Check sheet for the modelled part. Datum: model origin and axes. Units: mm. A direction names the side the tool comes from. Coordinates: 2 decimals unless noted, no trailing zeros. Loops run counter-clockwise (first coordinate to the right, second up) from the corner with the lowest first, then second, coordinate; pieces in that order, holes last. Notation, with made-up numbers: M 47,52 L 94,52 A12 cw 94,56 Z; hole C 41,21 d10. An arc over 180 degrees is marked long. Use CSV: the item, a comma, the result in double quotes. Start each with the question number.
(1) Section check C-C on y = -7.5. Record the cut outline in (x, z), and give its area (3 significant figures).
(2) Section check B-B on z = 33.5. Record the cut outline in (x, y), and give its area (3 significant figures).
(3) Set-up check for faces 1 (the flat face through (-105, -25.4, 26)), 2 (the flat face through (-90.02, -50.98, 14.5)), 3 (the flat face through (-2, -63.5, 15)): record each of +Z, -Z, +X, -X, +Y, -Y from which the full face is reachable in a straight line by a thin tool's end or side.
(4) Scan lines: line 1 (Y direction, x = -68, z = 31); line 2 (X direction, y = -41, z = 22.5); line 3 (X direction, y = -54.5, z = 24). Record each from-to range of solid material in increasing order.
(5) Section check A-A on x = -65. Record the cut outline in (y, z).
(6) Go/stop test with flat-tipped pins: pin 1 Ø1.5 at (x, z) = (-30.5, 15.5) entering from +Y; pin 2 Ø8 at (x, y) = (-94, -9) entering from +Z. Record where each tip stops, or that it passes through.
from build123d import *

# Parameters (mm, degrees)
F0_W     = 203.2
F0_H     = 50.8
F1_DEPTH = 63.5
F3_DEPTH = 25.4
F5_DEPTH = 25.4


with BuildPart() as f1:
    # F0 (on Front) → F1 (new body)
    with BuildSketch(Plane.XZ):
        with Locations((-22.86, 14.851971)):
            Rectangle(F0_W, F0_H)
    extrude(amount=F1_DEPTH)

    # F2 (on face) → F3 (cut)
    with BuildSketch(Plane.XZ.offset(63.5)):
        Polygon((-124.46, 40.251971), (-124.46, -10.548029), (-54.61, 40.251971), align=None)
    extrude(amount=-F3_DEPTH, mode=Mode.SUBTRACT)

    # F4 (on face) → F5 (cut)
    with BuildSketch(Plane(origin=(0, 0, 0), x_dir=(-1, 0, 0), z_dir=(0, 1, 0))):
        Polygon((54.61, 40.251971), (124.46, -10.548029), (124.46, 40.251971), align=None)
    extrude(amount=-F5_DEPTH, mode=Mode.SUBTRACT)


solid = f1.part
Outcome:
1,outline,"M -124.46,-10.55 L 78.74,-10.55 L 78.74,40.25 L -54.61,40.25 Z"
1,area,"8,550 mm²"
2,outline,"M -124.46,-38.1 L -63.89,-38.1 L -63.89,-63.5 L 78.74,-63.5 L 78.74,0 L -63.89,0 L -63.89,-25.4 L -124.46,-25.4 Z"
2,area,"9,830 mm²"
3,face 1,"+Z, -X, +Y"
3,face 2,"+Z, -X, -Y"
3,face 3,"+Z, -Z, +X, -X, -Y"
4,line 1,"y = -38.1 to -25.4"
4,line 2,"x = -79.02 to 78.74"
4,line 3,"x = -76.96 to 78.74"
5,outline,"M -63.5,-10.55 L 0,-10.55 L 0,32.7 L -25.4,32.7 L -25.4,40.25 L -38.1,40.25 L -38.1,32.7 L -63.5,32.7 Z"
6,pin 1,"stops at y = 0"
6,pin 2,"stops at z = 14.51"
